Check sheet for the modelled part. Datum: model origin and axes. Units: mm. Round coordinates to 2 decimals unless told otherwise and drop trailing zeros. One line per item, written item: value.
from build123d import *

# Parameters (mm, degrees)
F0_R     = 42.1386103745
F1_DEPTH = 76.2
F2_R     = 38.1
F3_R     = 38.09999


# Not quite as in the source:
# - a fillet or chamfer is up to 0.001 mm smaller than in the source, because OpenCascade refuses the exact size


with BuildPart() as f1:
    # F0 (on Front) → F1 (new body)
    with BuildSketch(Plane.XZ):
        Circle(F0_R)
    extrude(amount=F1_DEPTH)

    # F2
    f2_edges = [f1.edges().sort_by_distance(p)[0] for p in [
        (-42.13861, -76.2, 0),
    ]]
    fillet(f2_edges, radius=F2_R)

    # F3 (radius 38.1 in the source; OpenCascade refuses exactly that, so slightly less here)
    f3_edges = [f1.edges().sort_by_distance(p)[0] for p in [
        (42.13861, -19.05, 0),
        (-42.13861, -38.1, 0),
        (-42.13861, 0, 0),
    ]]
    fillet(f3_edges, radius=F3_R)


solid = f1.part
Item 1: Depth check by flat-ended pin: P1, Ø8, axis at x = -5, y = -20, coming from the -Z side; P2, Ø8, axis at x = 13.5, z = -27, coming from the +Y side; P3, Ø4, axis at x = 14.5, z = 4, coming from the +Y side. Enter the tip coordinate at first touch or a pass-through.
Answer:
P1: stops at z = -39.18
P2: stops at y = -7.1
P3: stops at y = -1.08
Item 2: Mould release check, pull along Y, two halves, no side actions. Record for faces 1 (the flat face through (0, 0, 0)), 2 (the flat face through (0, -76.2, 0)): pulls with the +Y half, pulls with the -Y half, needs draft (parallel to the pull), parting line crosses it, or undercut.
Answer:
face 1: pulls with the +Y half
face 2: pulls with the -Y half
Item 3: Thickness scan on line 1 (Z direction, x = -38, y = -42); line 2 (X direction, y = -33, z = 31); line 3 (X direction, y = -34.5, z = 32.5). Record the ranges inside material, lowest first.
Answer:
line 1: z = -17.74 to 17.74
line 2: x = -28.03 to 28.03
line 3: x = -26.55 to 26.55
